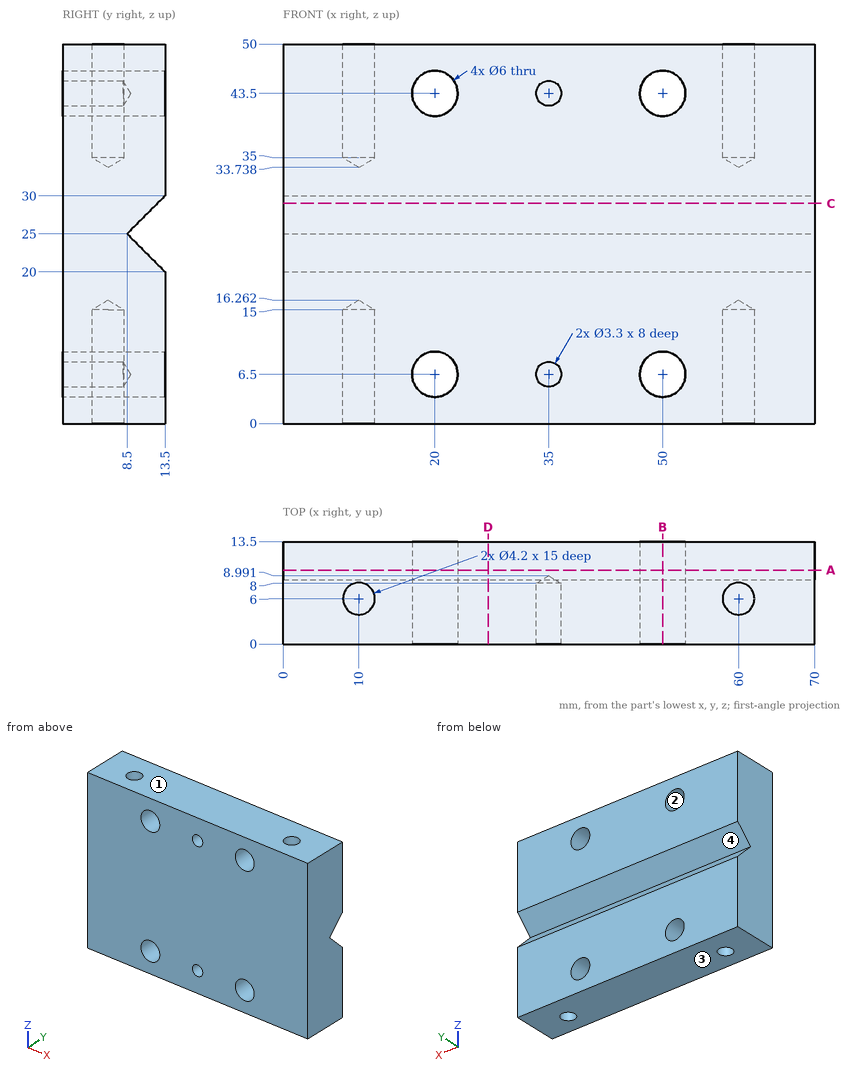
Geometry: see drawing. Coordinates: mm, zero at the bounding-box minimum. Round coordinates to 2 decimals unless told otherwise and drop trailing zeros. Loops run counter-clockwise (first coordinate to the right, second up) from the corner with the lowest first, then second, coordinate; pieces in that order, holes last. Notation, with made-up numbers: (37.5, -8) -> (73.5, -8) arc R20 cw to (73.5, -1) -> close; hole circle Ø11 at (65.25, 64). An arc over 180 degrees is marked (long way). One line per question, with ' | ' between items. Start each with the question number.
1. Section D-D on x = 27. Output: boundary loops of the cut face in (y, z), and give its area (3 significant figures).
2. Line query: line 1 along X through (y, z) = (10.5, 43.5); line 2 along Z through (x, y) = (50, 4); line 3 along X through (y, z) = (1.75, 6.5). Output: solid intervals per line, ascending. Write a range as [from, to].
3. Section C-C on z = 29. Output: boundary loops of the cut face in (x, y), and give its area (3 significant figures).
4. Section A-A on y = 9.75. Output: boundary loops of the cut face in (x, z).
5. Section B-B on x = 50. Output: boundary loops of the cut face in (y, z), and give its area (3 significant figures).
6. Mould query, pull axis Z, two halves, no side actions, for the marked faces 1, 2, 3 and 4. Classes: pulls with the +Z half, pulls with the -Z half, needs draft (parallel to the pull), parting line crosses it, or undercut.
7. Contact query for flat-ended pins moving along their axis: pin 1 (3.5 mm diameter, centred on x = 60, y = 6, fed in from -Z); pin 2 (3 mm diameter, centred on x = 35, z = 43.5, fed in from -Y). Output: stop coordinate, or through.
Returned:
1) outline: (0, 0) -> (13.5, 0) -> (13.5, 20) -> (8.5, 25) -> (13.5, 30) -> (13.5, 50) -> (0, 50) -> close | area: 650 mm2
2) line 1: x = [0, 17], [23, 47], [53, 70] | line 2: z = [0, 3.5], [9.5, 40.5], [46.5, 50] | line 3: x = [0, 17], [23, 33.35], [36.65, 47], [53, 70]
3) outline: (0, 0) -> (70, 0) -> (70, 12.5) -> (0, 12.5) -> close | area: 875 mm2
4) outline: (0, 0) -> (70, 0) -> (70, 23.75) -> (0, 23.75) -> close; (0, 26.25) -> (70, 26.25) -> (70, 50) -> (0, 50) -> close; hole circle Ø6 at (20, 6.5); hole circle Ø6 at (20, 43.5); hole circle Ø6 at (50, 6.5); hole circle Ø6 at (50, 43.5)
5) outline: (0, 0) -> (13.5, 0) -> (13.5, 3.5) -> (0, 3.5) -> close; (0, 9.5) -> (13.5, 9.5) -> (13.5, 20) -> (8.5, 25) -> (13.5, 30) -> (13.5, 40.5) -> (0, 40.5) -> close; (0, 46.5) -> (13.5, 46.5) -> (13.5, 50) -> (0, 50) -> close | area: 488 mm2
6) face 1: pulls with the +Z half | face 2: undercut | face 3: pulls with the -Z half | face 4: undercut
7) pin 1: stops at z = 15.21 | pin 2: stops at y = 8.09
